```python
from build123d import *

# Parameters (mm, degrees)
STREKKPR_VE_DEPTH = 1
FILLET1_R         = 12.5


with BuildPart() as part:
    # Sketch1 → Strekkprøve (new, symmetric)
    with BuildSketch(Plane.XY):
        with BuildLine():
            Line((2, -12.5), (2, 12.5))
            ThreePointArc((2, 12.5), (3.1443454, 16.623105626), (6.25, 19.566647013))
            Line((6.25, 19.566647013), (6.25, 37.5))
            Line((6.25, 37.5), (-6.25, 37.5))
            Line((-6.25, 37.5), (-6.25, 19.566647013))
            ThreePointArc((-6.25, 19.566647013), (-3.1443454, 16.623105626), (-2, 12.5))
            Line((-2, 12.5), (-2, -12.5))
            ThreePointArc((-2, -12.5), (-3.1443454, -16.623105626), (-6.25, -19.566647013))
            Line((-6.25, -19.566647013), (-6.25, -37.5))
            Line((-6.25, -37.5), (6.25, -37.5))
            Line((6.25, -37.5), (6.25, -19.566647013))
            ThreePointArc((6.25, -19.566647013), (3.1443454, -16.623105626), (2, -12.5))
        make_face()
    extrude(amount=STREKKPR_VE_DEPTH, both=True)

    # Fillet1
    fillet1_edges = [part.edges().sort_by_distance(p)[0] for p in [
        (6.25, -19.566647013, 0),
        (-6.25, -19.566647013, 0),
        (-6.25, 19.566647013, 0),
        (6.25, 19.566647013, 0),
    ]]
    fillet(fillet1_edges, radius=FILLET1_R)


solid = part.part
```
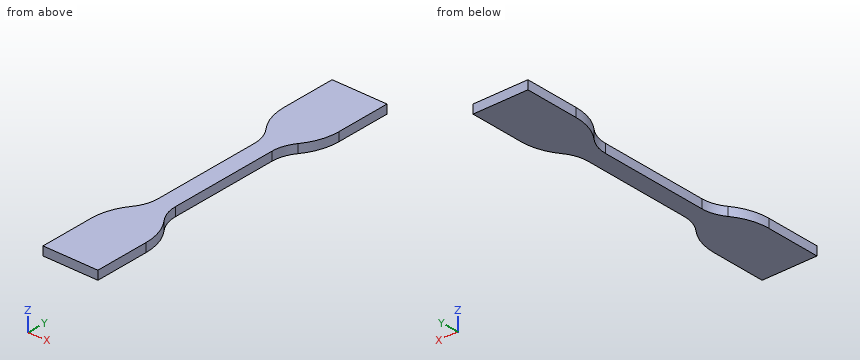
Part model, mm, in its own coordinate system. Round coordinates to 2 decimals unless told otherwise and drop trailing zeros. Loops run counter-clockwise (first coordinate to the right, second up) from the corner with the lowest first, then second, coordinate; pieces in that order, holes last.
1. Drill centre lines: line 1 along Y through (x, z) = (4.25, 0.95); line 2 along Y through (x, z) = (5, -0.9); line 3 along X through (y, z) = (11.5, 0.35). Where is each one in solid material? Low to high.
Solutions:
line 1: y = -37.5 to -18.22, 18.22 to 37.5
line 2: y = -37.5 to -19.55, 19.55 to 37.5
line 3: x = -2 to 2
2. Slice it at C-C (y = -5). Give the cut face in (x, z).
Solutions:
outline: (-2, -1) - (2, -1) - (2, 1) - (-2, 1) - close
3. Slice it at D-D (x = -2.75). Give the cut face in (y, z), and give its area (3 significant figures).
Solutions:
outline: (-37.5, -1) - (-15.88, -1) - (-15.88, 1) - (-37.5, 1) - close; (15.88, -1) - (37.5, -1) - (37.5, 1) - (15.88, 1) - close
area: 86.5 mm2
4. Flat gauge pins, fed straight in: pin 1 (1 mm diameter, centred on y = -3.5, z = -0.5, fed in from -X); pin 2 (1 mm diameter, centred on y = 15.5, z = 0.5, fed in from -X). Where does each tip first touch, or does it go through?
Solutions:
pin 1: stops at x = -2
pin 2: stops at x = -2.81
5. Slice it at A-A (x = 4.75). Give the cut face in (y, z).
Solutions:
outline: (-37.5, -1) - (-19.06, -1) - (-19.06, 1) - (-37.5, 1) - close; (19.06, -1) - (37.5, -1) - (37.5, 1) - (19.06, 1) - close
6. Slice it at B-B (z = -0.3). Give the cut face in (x, y).
Solutions:
outline: (-6.25, -37.5) - (6.25, -37.5) - (6.25, -25) arc R12.5 ccw to (3.66, -17.38) arc R8 cw to (2, -12.5) - (2, 12.5) arc R8 cw to (3.66, 17.38) arc R12.5 ccw to (6.25, 25) - (6.25, 37.5) - (-6.25, 37.5) - (-6.25, 25) arc R12.5 ccw to (-3.66, 17.38) arc R8 cw to (-2, 12.5) - (-2, -12.5) arc R8 cw to (-3.66, -17.38) arc R12.5 ccw to (-6.25, -25) - close
